```python
from build123d import *

# Parameters (mm, degrees)
SKETCH1_W           = 48.25
SKETCH1_H           = 27.65
SKETCH1_W_2         = 45.25
SKETCH1_H_2         = 24.65
MAIN_BODY_DEPTH     = 4
SKETCH3_W           = 45.25
SKETCH3_H           = 24.65
SKETCH3_W_2         = 42.25
SKETCH3_H_2         = 21.65
BOSS_EXTRUDE2_DEPTH = 2.6
BOSS_EXTRUDE3_START = -2.6
BOSS_EXTRUDE3_DEPTH = 4
SKETCH5_R           = 1.075
CUT_EXTRUDE1_DEPTH  = 1.4
SKETCH6_R           = 1.075
CUT_EXTRUDE2_DEPTH  = 3.6
FILLET1_R           = 2


with BuildPart() as part:
    # Sketch1 → Main Body (new body)
    with BuildSketch(Plane.XY):
        with Locations((22.625, 12.325)):
            Rectangle(SKETCH1_W, SKETCH1_H)
        with Locations((22.625, 12.325)):
            Rectangle(SKETCH1_W_2, SKETCH1_H_2, mode=Mode.SUBTRACT)
    extrude(amount=MAIN_BODY_DEPTH)

    # Sketch3 → Boss-Extrude2 (add)
    with BuildSketch(Plane.XY.offset(4)):
        with Locations((22.625, 12.325)):
            Rectangle(SKETCH3_W, SKETCH3_H)
        with Locations((22.625, 12.325)):
            Rectangle(SKETCH3_W_2, SKETCH3_H_2, mode=Mode.SUBTRACT)
    extrude(amount=-BOSS_EXTRUDE2_DEPTH)

    # Sketch4 → Boss-Extrude3 (add)
    with BuildSketch(Plane(origin=(0, 0, 1.4), x_dir=(-1, 0, 0), z_dir=(0, 0, -1)).offset(BOSS_EXTRUDE3_START)):
        with BuildLine():
            Line((-1.125, 21.575), (-1.125, 23.575))
            Line((-1.125, 23.575), (-3.125, 23.575))
            ThreePointArc((-3.125, 23.575), (-4.539213562, 20.160786438), (-1.125, 21.575))
        make_face()
        with BuildLine():
            Line((-1.125, 1.075), (-3.125, 1.075))
            ThreePointArc((-3.125, 1.075), (-4.539213562, 4.489213562), (-1.125, 3.075))
            Line((-1.125, 3.075), (-1.125, 1.075))
        make_face()
        with BuildLine():
            Line((-44.125, 3.075), (-44.125, 1.075))
            Line((-44.125, 1.075), (-42.125, 1.075))
            ThreePointArc((-42.125, 1.075), (-40.710786438, 4.489213562), (-44.125, 3.075))
        make_face()
        with BuildLine():
            Line((-44.125, 23.575), (-42.125, 23.575))
            ThreePointArc((-42.125, 23.575), (-40.710786438, 20.160786438), (-44.125, 21.575))
            Line((-44.125, 21.575), (-44.125, 23.575))
        make_face()
    extrude(amount=BOSS_EXTRUDE3_DEPTH)

    # Sketch5 → Cut-Extrude1 (cut)
    with BuildSketch(Plane(origin=(0, 0, 0), x_dir=(-1, 0, 0), z_dir=(0, 0, -1))):
        with BuildLine():
            ThreePointArc((-1.125, 21.575), (-1.710786438, 22.989213562), (-3.125, 23.575))
            Line((-3.125, 23.575), (-1.125, 23.575))
            Line((-1.125, 23.575), (-1.125, 21.575))
        make_face()
        with Locations((-3.125, 21.575)):
            Circle(SKETCH5_R)
        with Locations((-3.125, 3.075)):
            Circle(SKETCH5_R)
        with BuildLine():
            Line((-1.125, 1.075), (-1.125, 3.075))
            ThreePointArc((-1.125, 3.075), (-1.710786438, 1.660786438), (-3.125, 1.075))
            Line((-3.125, 1.075), (-1.125, 1.075))
        make_face()
        with Locations((-42.125, 3.075)):
            Circle(SKETCH5_R)
        with BuildLine():
            ThreePointArc((-44.125, 3.075), (-43.539213562, 1.660786438), (-42.125, 1.075))
            Line((-42.125, 1.075), (-44.125, 1.075))
            Line((-44.125, 1.075), (-44.125, 3.075))
        make_face()
        with Locations((-42.125, 21.575)):
            Circle(SKETCH5_R)
        with BuildLine():
            ThreePointArc((-42.125, 23.575), (-43.539213562, 22.989213562), (-44.125, 21.575))
            Line((-44.125, 21.575), (-44.125, 23.575))
            Line((-44.125, 23.575), (-42.125, 23.575))
        make_face()
    extrude(amount=-CUT_EXTRUDE1_DEPTH, mode=Mode.SUBTRACT)

    # Sketch6 → Cut-Extrude2 (cut, through all)
    with BuildSketch(Plane(origin=(0, 0, 1.4), x_dir=(-1, 0, 0), z_dir=(0, 0, -1))):
        with Locations((-3.125, 21.575)):
            Circle(SKETCH6_R)
        with Locations((-3.125, 3.075)):
            Circle(SKETCH6_R)
        with Locations((-42.125, 3.075)):
            Circle(SKETCH6_R)
        with Locations((-42.125, 21.575)):
            Circle(SKETCH6_R)
    extrude(amount=-CUT_EXTRUDE2_DEPTH, mode=Mode.SUBTRACT)

    # Fillet1
    fillet1_edges = [part.edges().sort_by_distance(p)[0] for p in [
        (43.75, 20.409077618, 2.7),
        (40.892370696, 23.15, 2.7),
        (45.25, 24.65, 0.7),
        (0, 24.65, 0.7),
        (45.25, 0, 0.7),
        (0, 0, 0.7),
        (4.357629304, 1.5, 2.7),
        (1.5, 4.240922382, 2.7),
        (43.75, 4.240922382, 2.7),
        (-1.5, 26.15, 2),
        (46.75, 26.15, 2),
        (40.892370696, 1.5, 2.7),
        (46.75, -1.5, 2),
        (-1.5, -1.5, 2),
        (4.357629304, 23.15, 2.7),
        (1.5, 20.409077618, 2.7),
    ]]
    fillet(fillet1_edges, radius=FILLET1_R)


solid = part.part
```
Source: CAD feature listing. Evaluate the final solid. Frame: model axes, mm. A direction names the side the tool comes from. Give positions to 0.01 mm unless a question says otherwise; leave off trailing zeros. Loops run counter-clockwise (first coordinate to the right, second up) from the corner with the lowest first, then second, coordinate; pieces in that order, holes last. Notation, with made-up numbers: (5.25, 68.25) -> (58.25, 68.25) arc R27 ccw to (58.25, 98.25) -> close; hole circle Ø11 at (41, 8). An arc over 180 degrees is marked (long way). Use a Markdown table: item, result. Add a question column.
(1) Pull-direction query (X, two-part tool) for faces 1 (the face through (41, 2, 0)), 2 (the face through (22, 23.15, 3)), 3 (the face through (-0.9, 25.58, 2.03)), 4 (the face through (44.65, 24.08, 0.71)); classes: +X half, -X half, draft (parallel to the pull), parting line (faces both ways), or undercut.
(2) Access query for faces 5 (the face through (43.75, 12, 3)), 6 (the face through (44.68, 0.6, 0.71)), 7 (the face through (46.18, 25.55, 2.03)). Directions: +Z, -Z, +X, -X, +Y, -Y. A direction counts if a zero-diameter tool reaches every point of the face in a straight line with its end or side. Return the directions, or none.
(3) Section query C-C (y = 13). Output: boundary loops of the cut face in (x, z), then the cut area to 3 significant figures.
(4) Ray query, line 1 (Y direction, x = 19, z = 2.3); line 2 (X direction, y = 21.75, z = 0.75); line 3 (X direction, y = 7.75, z = 0.8). Return the intervals inside material, ascending.
(5) Section query A-A (x = 23). Output: boundary loops of the cut face in (y, z), then the cut area to 3 significant figures.
(6) Section query B-B (z = 0.5). Count the separate pieces of the cut face and the enclosed holes in it, then the cut area to 3 significant figures.
(7) Section query D-D (y = 2.5). Output: boundary loops of the cut face in (x, z).
Checked values:
| question | item | result |
|---|---|---|
| 1 | face 1 | draft |
| 1 | face 2 | undercut |
| 1 | face 3 | -X half |
| 1 | face 4 | undercut |
| 2 | face 5 | +Z, -Z |
| 2 | face 6 | -Z |
| 2 | face 7 | +Z, -Z, +X, +Y |
| 3 | outline | (-1.5, 0) -> (0, 0) -> (0, 1.4) -> (1.5, 1.4) -> (1.5, 4) -> (-1.5, 4) -> close; (43.75, 1.4) -> (45.25, 1.4) -> (45.25, 0) -> (46.75, 0) -> (46.75, 4) -> (43.75, 4) -> close |
| 3 | area | 19.8 mm^2 |
| 4 | line 1 | -1.5 to 1.5, 23.15 to 26.15 |
| 4 | line 2 | -1.5 to 0, 1.13 to 2.06, 4.19 to 5.12, 40.13 to 41.06, 43.19 to 44.12, 45.25 to 46.75 |
| 4 | line 3 | -1.5 to 0, 45.25 to 46.75 |
| 5 | outline | (-1.5, 0) -> (0, 0) -> (0, 1.4) -> (1.5, 1.4) -> (1.5, 4) -> (-1.5, 4) -> close; (23.15, 1.4) -> (24.65, 1.4) -> (24.65, 0) -> (26.15, 0) -> (26.15, 4) -> (23.15, 4) -> close |
| 5 | area | 19.8 mm^2 |
| 6 | separate pieces | 5 |
| 6 | enclosed holes | 5 |
| 6 | area | 254 mm^2 |
| 7 | outline | (-1.5, 0) -> (0, 0) -> (0, 1.4) -> (1.21, 1.4) -> (1.21, 0) -> (2.22, 0) -> (2.22, 4) -> (-1.5, 4) -> close; (4.03, 0) -> (5.04, 0) -> (5.04, 1.4) -> (5.37, 1.4) -> (5.37, 4) -> (4.03, 4) -> close; (39.88, 1.4) -> (40.21, 1.4) -> (40.21, 0) -> (41.22, 0) -> (41.22, 4) -> (39.88, 4) -> close; (43.03, 0) -> (44.04, 0) -> (44.04, 1.4) -> (45.25, 1.4) -> (45.25, 0) -> (46.75, 0) -> (46.75, 4) -> (43.03, 4) -> close |
